Check sheet for the modelled part. Datum: model origin and axes. Units: mm. Give positions to 0.01 mm unless a question says otherwise; leave off trailing zeros. Loops run counter-clockwise (first coordinate to the right, second up) from the corner with the lowest first, then second, coordinate; pieces in that order, holes last. Notation, with made-up numbers: (-27, -29.5) - (-12, -29.5) arc R14 cw to (-12, -7.5) - close; hole circle Ø4 at (31.25, -13.5). An arc over 180 degrees is marked (long way). Answer in a Markdown table with one row per item. Add a question column.
(1) Go/stop test with flat-tipped pins: P1, Ø1.5, axis at y = -2.5, z = 302.5, coming from the +X side; P2, Ø4, axis at x = -35, y = -3.5, coming from the +Z side; P3, Ø1, axis at x = -453.5, y = 4, coming from the -Z side. Record where each tip stops, or that it passes through.
(2) Sectioned sample at A-A on z = -746. Enter the section's corners in (x, y).
(3) Sectioned sample at B-B on x = -527.5. Enter the section's corners in (y, z).
(4) Thickness scan on L1, parallel to Z at x = 0, y = 1.5; L2, parallel to Y at x = -379, z = 404; L3, parallel to X at y = 2.5, z = -4.5. Record the ranges inside material, lowest first.
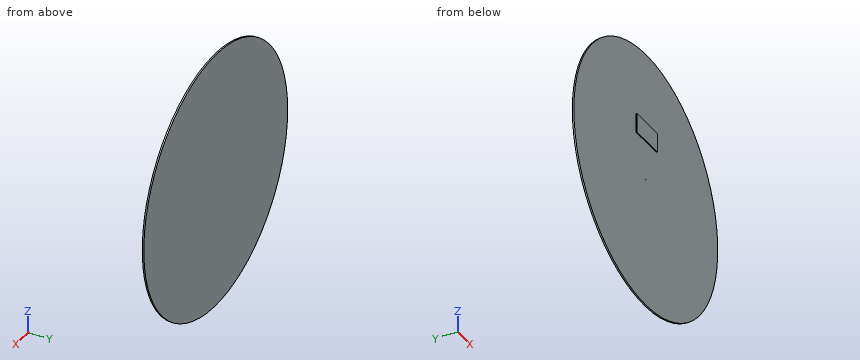
Autodesk Inventor part; units mm, degrees
ref_plane "YZ Plane" through (0, 0, 0) normal (1, 0, 0) x (0, 1, 0)
ref_plane "XZ Plane" through (0, 0, 0) normal (0, 1, 0) x (-1, 0, 0)
ref_plane "XY Plane" through (0, 0, 0) normal (0, 0, 1) x (1, 0, 0)
sketch "Sketch1" plane through (0, 0, 0) normal (0, 1, 0) x (-1, 0, 0)
  circle A0 centre (0, 0) radius 850
  dimension "d0" = 1700
extrude "Extrusion1" add sketch "Sketch1" along normal blind 10
sketch "Sketch2" plane through (0, 0, 0) normal (0, -1, 0) x (1, 0, 0)
  circle A0 centre (0, 0) radius 2.5
  dimension "d3" = 5
extrude "Extrusion2" cut sketch "Sketch2" against normal blind 5
sketch "Sketch3" plane through (0, 0, 0) normal (0, -1, 0) x (1, 0, 0)
  line L0 (-114.2279, 383.8588) -> (126.182, 383.8588)
  line L1 (126.182, 383.8588) -> (126.182, 257.6769)
  line L2 (126.182, 257.6769) -> (-114.2279, 257.6769)
  line L3 (-114.2279, 257.6769) -> (-114.2279, 383.8588)
  point P0 (0, 0)
extrude "Extrusion3" add sketch "Sketch3" along normal blind 5
properties part number "McCrea_ukruhlaPlocha_walle" material "Rubber"
Reply:
| question | item | result |
|---|---|---|
| 1 | P1 | x = 126.18 |
| 1 | P2 | z = 383.86 |
| 1 | P3 | z = -719.23 |
| 2 | outline | (-407.41, 0) - (407.41, 0) - (407.41, 10) - (-407.41, 10) - close |
| 3 | outline | (0, -666.52) - (10, -666.52) - (10, 666.52) - (0, 666.52) - close |
| 4 | L1 | -850 to -2.5, 2.5 to 850 |
| 4 | L2 | 0 to 10 |
| 4 | L3 | -849.99 to 849.99 |
